Read the model definition and answer for the solid it produces. Units are mm, in the model's axes. A direction names the side the tool comes from. Give positions to 0.01 mm unless a question says otherwise; leave off trailing zeros. Order: outer loops, then holes, each group sorted by start corner. A loop starts at its lowest first (then second) coordinate and runs counter-clockwise, first axis right, second up.
Item 1: A cutting plane is placed at B-B (z = 0). Write down the section's boundary in (x, y).
Item 2: Given pin 1 Ø1 at (x, z) = (-17.5, -5.5) entering from -Y; pin 2 Ø12 at (x, y) = (10, -12) entering from +Z; pin 3 Ø5 at (y, z) = (-63, -10) entering from +X; pin 4 Ø3 at (x, z) = (0.5, -20) entering from +Y, each flat-ended and moving along its own axis, determine where each tip first touches the part or whether it passes through.
Item 3: A cutting plane is placed at D-D (y = -70.5). Write down the section's boundary in (x, z), plus the area to 3 significant figures.
Item 4: Which of the six approach directions +Z, -Z, +X, -X, +Y, -Y give full straight-line access (tool end or side, diameter ignored) to faces 1 (the face through (14, -25.4, 8)), 2 (the face through (0, -76.2, 0))?
Item 5: A cutting plane is placed at A-A (x = 0). Write down the section's boundary in (y, z), plus the area to 3 significant figures.
Item 6: A cutting plane is placed at C-C (y = -9). Write down the section's boundary in (x, z), plus the area to 3 significant figures.
Item 7: Find the intervals of material crossed by line 1 along X through (y, z) = (-61, -0.5); line 2 along Y through (x, z) = (-12.5, 29); line 3 along Z through (x, y) = (-7, -24), in increasing order.
from build123d import *

# Parameters (mm, degrees)
F0_R     = 32.34451
F1_DEPTH = 25.4
F2_R     = 15.47955
F3_DEPTH = 76.2
F4_R     = 8.094694
F5_DEPTH = 25.4


with BuildPart() as f1:
    # F0 (on Front) → F1 (new body)
    with BuildSketch(Plane.XZ):
        Circle(F0_R)
    extrude(amount=F1_DEPTH)

    # F2 (on Front) → F3 (join)
    with BuildSketch(Plane.XZ):
        Circle(F2_R)
    extrude(amount=F3_DEPTH)

    # F4 (on Front) → F5 (cut)
    with BuildSketch(Plane.XZ):
        Circle(F4_R)
    extrude(amount=-F5_DEPTH, mode=Mode.SUBTRACT)


solid = f1.part
Response values:
1. outline: (-32.34, -25.4) - (-15.48, -25.4) - (-15.48, -76.2) - (15.48, -76.2) - (15.48, -25.4) - (32.34, -25.4) - (32.34, 0) - (-32.34, 0) - close
2. pin 1: stops at y = -25.4
2. pin 2: stops at z = 32.1
2. pin 3: stops at x = 13.54
2. pin 4: stops at y = 0
3. outline: circle Ø30.96 at (0, 0)
3. area: 753 mm2
4. face 1: -Y
4. face 2: +Z, -Z, +X, -X, -Y
5. outline: (-76.2, -15.48) - (-25.4, -15.48) - (-25.4, -32.34) - (0, -32.34) - (0, 32.34) - (-25.4, 32.34) - (-25.4, 15.48) - (-76.2, 15.48) - close
5. area: 3,220 mm2
6. outline: circle Ø64.69 at (0, 0)
6. area: 3,290 mm2
7. line 1: x = -15.47 to 15.47
7. line 2: y = -25.4 to 0
7. line 3: z = -31.58 to 31.58
